Verification items for the finished model (mm, model axes). Round coordinates to 2 decimals unless told otherwise and drop trailing zeros. Write each loop counter-clockwise with the first axis right and the second up, starting at its lowest first coordinate (ties: lowest second). Pieces come first, ordered by that corner, then holes. Notation, with made-up numbers: (-21.5, -7) - (34.5, -7) arc R17 cw to (34.5, 8) - close; hole circle Ø3 at (58, -37.75). An arc over 180 degrees is marked (long way). Write each question's results on one line, items separated by ' | '.
```python
from build123d import *

# Parameters (mm, degrees)
AXIAL_PROFILE_MM_W     = 4
AXIAL_PROFILE_MM_H     = 47
AXIAL_HOLES_DEPTH      = 152.492574075
AXIAL_HOLES_DEPTH_BACK = 152.492574075
SKETCH2_R              = 1.65


with BuildPart() as part:
    # Axial profile (mm) → Full revolution (revolve)
    with BuildSketch(Plane.XY, mode=Mode.PRIVATE) as full_revolution_sk:
        with Locations((-128, 31.5)):
            Rectangle(AXIAL_PROFILE_MM_W, AXIAL_PROFILE_MM_H)
    revolve(full_revolution_sk.sketch.rotate(Axis((-110, 0, 0), (1, 0, 0)), 90), axis=Axis((-110, 0, 0), (1, 0, 0)))

    # Sketch2 → Axial holes (cut, two sides: drawn at the far end of the back side and taken through both)
    with BuildSketch(Plane(origin=(0, 0, 0), x_dir=(0, 0, -1), z_dir=(1, 0, 0)).offset(-AXIAL_HOLES_DEPTH_BACK)):
        with Locations((0, 52)):
            Circle(SKETCH2_R)
        with Locations((-52, 0)):
            Circle(SKETCH2_R)
        with Locations((0, -52)):
            Circle(SKETCH2_R)
        with Locations((52, 0)):
            Circle(SKETCH2_R)
    extrude(amount=AXIAL_HOLES_DEPTH + AXIAL_HOLES_DEPTH_BACK, mode=Mode.SUBTRACT)


solid = part.part
```
(1) Section check B-B (z = 52). Record the cut outline in (x, y), plus the area to 3 significant figures.
Answer:
outline: (-130, -17.92) - (-126, -17.92) - (-126, -1.65) - (-130, -1.65) - close; (-130, 1.65) - (-126, 1.65) - (-126, 17.92) - (-130, 17.92) - close | area: 130 mm2
(2) Thickness scan on L1, parallel to Y at x = -128.2, z = 0; L2, parallel to Z at x = -126.85, y = 42; L3, parallel to Z at x = -126.6, y = -39.5. Record the ranges inside material, lowest first.
Answer:
L1: -55 to -53.65, -50.35 to -8, 8 to 50.35, 53.65 to 55 | L2: -35.51 to 35.51 | L3: -38.27 to 38.27
(3) Mould release check, pull along Z, two halves, no side actions. Record for faces 1 (the cylindrical face through (-128.03, 53.39, -0.89)), 2 (the cylindrical face through (-127.972, 48.794, 25.379)), 3 (the flat face through (-126, 11, 1)): released by +Z, released by -Z, zero draft, split by the parting line, or undercut.
Answer:
face 1: undercut | face 2: split by the parting line | face 3: zero draft
(4) Go/stop test with flat-tipped pins: pin 1 Ø1 at (x, y) = (-128.5, -32) entering from +Z; pin 2 Ø1.5 at (x, y) = (-127.5, 32.5) entering from -Z; pin 3 Ø1.5 at (x, y) = (-126.5, 12) entering from -Z. Record where each tip stops, or that it passes through.
Answer:
pin 1: z = 45.09 | pin 2: z = -44.91 | pin 3: z = -53.84
(5) Section check C-C (x = -128.9). Record the cut outline in (y, z).
Answer:
outline: circle Ø110 at (0, 0); hole circle Ø3.3 at (-52, 0); hole circle Ø16 at (0, 0); hole circle Ø3.3 at (0, -52); hole circle Ø3.3 at (0, 52); hole circle Ø3.3 at (52, 0)
(6) Section check A-A (z = 0). Record the cut outline in (x, y).
Answer:
outline: (-130, -55) - (-126, -55) - (-126, -53.65) - (-130, -53.65) - close; (-130, -50.35) - (-126, -50.35) - (-126, -8) - (-130, -8) - close; (-130, 8) - (-126, 8) - (-126, 50.35) - (-130, 50.35) - close; (-130, 53.65) - (-126, 53.65) - (-126, 55) - (-130, 55) - close
